Work out the finished part from the listing and answer in its coordinate system (mm). Face numbers are marked on the shaded views. Coordinates: 2 decimals unless noted, no trailing zeros. Write each loop counter-clockwise with the first axis right and the second up, starting at its lowest first coordinate (ties: lowest second). Pieces come first, ordered by that corner, then holes. Notation, with made-up numbers: (-7.5, -16) - (25.5, -16) arc R9 ccw to (25.5, 0) - close; hole circle Ø11 at (5.25, 54.5). An arc over 180 degrees is marked (long way). Use a Markdown table: item, result. Add a question column.
(1) Given pin 1 Ø10 at (x, z) = (-22, -100) entering from +Y; pin 2 Ø3 at (x, z) = (-26.5, -76) entering from +Y; pin 3 Ø10 at (y, z) = (27, -51) entering from -X, each flat-ended and moving along its own axis, determine where each tip first touches the part or whether it passes through.
(2) The part is cut by section C-C, the plane z = -93. Give the vertices of the cut face in (x, y).
(3) For a pull along Y with two mould halves and no side action, classify the marked faces 1, 2 and 3 as released by +Y, released by -Y, zero draft, split by the parting line, or undercut.
(4) Find the intervals of material crossed by line 1 (X direction, y = -21.5, z = -133); line 2 (Y direction, x = 13.5, z = -91); line 3 (Y direction, x = 20.5, z = -73.5), in increasing order. Write a range as from..to.
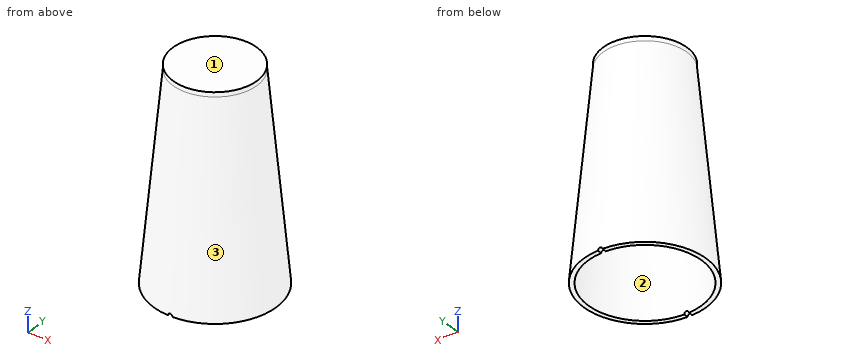
from build123d import *

# Parameters (mm, degrees)
SHELL3_T                = -3.175
SKETCH5_R               = 29.36875
BOSS_EXTRUDE1_DEPTH     = 3.175
FILLET1_R               = 3.175
CUT_EXTRUDE1_DEPTH      = 156.201976268
CUT_EXTRUDE1_DEPTH_BACK = 156.201976268
SKETCH6_R               = 1.5875


with BuildPart() as part:
    # Sketch2 → Revolve1 (revolve)
    with BuildSketch(Plane(origin=(0, 0, 0), x_dir=(1, 0, 0), z_dir=(0, 1, 0))):
        Polygon((29.36875, 0), (0, 0), (0, 142.875), (42.8625, 142.875), align=None)
    revolve(axis=Axis((0, 0, 0), (0, 0, -1)))

    # Shell3
    shell3_openings = [part.faces().sort_by_distance(p)[0] for p in [
        (0, 0, -142.875),
    ]]
    offset(amount=SHELL3_T, openings=shell3_openings, kind=Kind.INTERSECTION)

    # Sketch5 → Boss-Extrude1 (add)
    with BuildSketch(Plane.XY):
        Circle(SKETCH5_R)
    extrude(amount=BOSS_EXTRUDE1_DEPTH)

    # Fillet1
    fillet1_edges = [part.edges().sort_by_distance(p)[0] for p in [
        (-26.479482439, 0, -3.175),
    ]]
    fillet(fillet1_edges, radius=FILLET1_R)

    # Sketch6 → Cut-Extrude1 (cut, two sides: drawn at the far end of the back side and taken through both)
    with BuildSketch(Plane(origin=(0, 0, 0), x_dir=(1, 0, 0), z_dir=(0, 1, 0)).offset(-CUT_EXTRUDE1_DEPTH_BACK)):
        with Locations((0, 142.875)):
            Circle(SKETCH6_R)
    extrude(amount=CUT_EXTRUDE1_DEPTH + CUT_EXTRUDE1_DEPTH_BACK, mode=Mode.SUBTRACT)


solid = part.part
Model answer:
| question | item | result |
|---|---|---|
| 1 | pin 1 | y = 34.95 |
| 1 | pin 2 | y = 26.67 |
| 1 | pin 3 | x = -26.21 |
| 2 | outline | circle Ø76.3 at (0, 0); hole circle Ø69.93 at (0, 0) |
| 3 | face 1 | zero draft |
| 3 | face 2 | undercut |
| 3 | face 3 | split by the parting line |
| 4 | line 1 | -36..-32.23, 32.23..36 |
| 4 | line 2 | -35.48..-32.05, 32.05..35.48 |
| 4 | line 3 | -29.97..-26.01, 26.01..29.97 |
